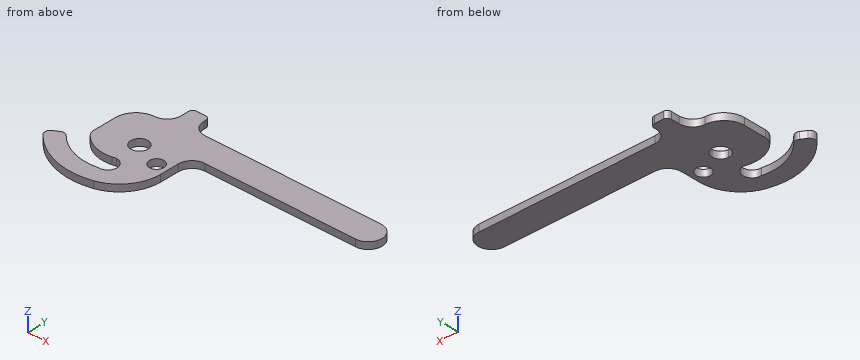
from build123d import *

# Parameters (mm, degrees)
F0_R     = 6.6675
F1_DEPTH = 6.35


with BuildPart() as f1:
    # F0 (on Top) → F1 (new body)
    with BuildSketch(Plane.XY):
        with BuildLine():
            ThreePointArc((0, -7.9375), (5.61266, -5.61266), (7.9375, 0))
            ThreePointArc((7.9375, 0), (-5.61266, 5.61266), (0, -7.9375))
        make_face()
        with BuildLine():
            ThreePointArc((-3.19381, -23.695523), (-1.627902, -23.2228), (0, -23.0632))
            ThreePointArc((0, -23.0632), (8.372137, -31.851707), (-0.812057, -39.787771))
            ThreePointArc((-0.812057, -39.787771), (-24.496198, -38.037618), (-44.408232, -25.094956))
            ThreePointArc((-44.408232, -25.094956), (-47.379559, -23.510637), (-50.688938, -24.132628))
            Line((-50.688938, -24.132628), (-55.635531, -26.988545))
            ThreePointArc((-55.635531, -26.988545), (-58.108455, -30.56516), (-56.908568, -34.744611))
            ThreePointArc((-56.908568, -34.744611), (-27.458308, -53.618524), (7.5184, -54.03359))
            ThreePointArc((7.5184, -54.03359), (27.748901, -40.39788), (35.56, -17.285276))
            Line((35.56, -17.285276), (35.56, 0))
            Line((35.56, 0), (35.56, 0.508))
            ThreePointArc((35.56, 0.508), (39.279744, 9.488256), (48.26, 13.208))
            Line((48.26, 13.208), (187.5028, 13.208))
            ThreePointArc((187.5028, 13.208), (200.2028, 25.908), (187.5028, 38.608))
            Line((187.5028, 38.608), (24.892, 38.608))
            ThreePointArc((24.892, 38.608), (15.911744, 42.327744), (12.192, 51.308))
            Line((12.192, 51.308), (12.192, 53.34))
            ThreePointArc((12.192, 53.34), (11.076077, 56.034077), (8.382, 57.15))
            Line((8.382, 57.15), (0, 57.15))
            ThreePointArc((0, 57.15), (-2.694077, 56.034077), (-3.81, 53.34))
            Line((-3.81, 53.34), (-3.81, 45.709836))
            ThreePointArc((-3.81, 45.709836), (-7.3519, 36.911018), (-16.002, 33.02))
            ThreePointArc((-16.002, 33.02), (-29.472384, 27.440384), (-35.052, 13.97))
            Line((-35.052, 13.97), (-35.052, -6.785096))
            ThreePointArc((-35.052, -6.785096), (-34.210819, -11.088793), (-31.811089, -14.759036))
            ThreePointArc((-31.811089, -14.759036), (-18.633931, -22.850619), (-3.19381, -23.695523))
        make_face()
        with BuildLine():
            ThreePointArc((0, -7.9375), (-5.61266, 5.61266), (7.9375, 0))
            ThreePointArc((7.9375, 0), (5.61266, -5.61266), (0, -7.9375))
        make_face(mode=Mode.SUBTRACT)
        with Locations((24.8666, -9.652)):
            Circle(F0_R, mode=Mode.SUBTRACT)
    extrude(amount=-F1_DEPTH)


solid = f1.part
Geometry check sheet. Reference: the model listing, model coordinates, mm. Give positions to 0.01 mm unless a question says otherwise; leave off trailing zeros. Write each loop counter-clockwise with the first axis right and the second up, starting at its lowest first coordinate (ties: lowest second). Pieces come first, ordered by that corner, then holes. Notation, with made-up numbers: (43.25, 72) - (70.25, 72) arc R15 cw to (70.25, 88) - close; hole circle Ø4 at (83.25, 19.5). An arc over 180 degrees is marked (long way). Put each result on its own line as item: value.
1. Sectioned sample at C-C, the plane x = 109. Enter the section's corners in (y, z).
Ans:
outline: (13.21, -6.35) - (38.61, -6.35) - (38.61, 0) - (13.21, 0) - close
2. Sectioned sample at D-D, the plane y = -43.5. Enter the section's corners in (x, z).
Ans:
outline: (-47.46, -6.35) - (25.11, -6.35) - (25.11, 0) - (-47.46, 0) - close
3. Sectioned sample at B-B, the plane z = -3.75. Give the number of separate pieces and of enclosed holes in the cut face, plus the area to 3 significant figures.
Ans:
separate pieces: 1
enclosed holes: 2
area: 9,880 mm²
4. Sectioned sample at A-A, the plane y = -31. Enter the section's corners in (x, z).
Ans:
outline: (-58.16, -6.35) - (-37.88, -6.35) - (-37.88, 0) - (-58.16, 0) - close; (8.37, -6.35) - (33.01, -6.35) - (33.01, 0) - (8.37, 0) - close
5. Go/stop test with flat-tipped pins: pin 1 (3 mm diameter, centred on x = 110, z = -4, fed in from +Y); pin 2 (3 mm diameter, centred on y = 50.5, z = -4, fed in from -X); pin 3 (2 mm diameter, centred on x = -24.5, z = -2, fed in from -Y). Record where each tip stops, or that it passes through.
Ans:
pin 1: stops at y = 38.61
pin 2: stops at x = -3.81
pin 3: stops at y = -54.67
6. Thickness scan on line 1 (Y direction, x = 92, z = -5.75); line 2 (Y direction, x = -23, z = -5.25); line 3 (Y direction, x = -13.5, z = -0.5). Record the ranges inside material, lowest first.
Ans:
line 1: y = 13.21 to 38.61
line 2: y = -54.78 to -38.51, -21.12 to 31.69
line 3: y = -56.14 to -40.35, -23.99 to 33.37
